Input: part model. Units: mm. Frame: model coordinates. A direction names the side the tool comes from. Give positions to 0.01 mm unless a question says otherwise; leave off trailing zeros. Loops run counter-clockwise (first coordinate to the right, second up) from the corner with the lowest first, then second, coordinate; pieces in that order, holes last. Notation, with made-up numbers: M 86,87 L 112,87 A12 cw 112,107 Z; hole C 17,21.25 d8. An arc over 180 degrees is marked long. Return JSON: item names as keys, results as strings. Group by question number.
```python
from build123d import *

# Parameters (mm, degrees)
CHAMFER1_SIZE                                    = 3.81
HOLE2_D                                          = 6
CIRPATTERN2_COUNT                                = 10
CBORE_FOR_1_4_SOCKET_SHOULDER_SCREW1_D           = 6.7564
CBORE_FOR_1_4_SOCKET_SHOULDER_SCREW1_CBORE_D     = 10.31748
CBORE_FOR_1_4_SOCKET_SHOULDER_SCREW1_CBORE_DEPTH = 4.7752
CIRPATTERN4_COUNT                                = 12
CUT_EXTRUDE3_REACH                               = 116.288
CIRPATTERN5_COUNT                                = 12


with BuildPart() as part:
    # Sketch1 → Revolve1 (revolve)
    with BuildSketch(Plane.XY):
        Polygon((79.375, 10.68578), (79.375, 17.03578), (13.52042, 17.03578), (13.52042, 25.13076), (9.71042, 25.13076), (9.71042, 0), (14.14526, -4.43484), (19.22526, -4.43484), (19.22526, 10.68578), align=None)
    revolve(axis=Axis((0, 0, 0), (0, 1, 0)))

    # Chamfer1
    chamfer1_edges = [part.edges().sort_by_distance(p)[0] for p in [
        (-13.52042, 25.13076, 0),
    ]]
    chamfer(chamfer1_edges, length=CHAMFER1_SIZE - 0.0001)  # a hair under: the kernel refuses the full size

    # Hole2 (through all)
    with Locations(Plane(origin=(0, 17.03578, 0), x_dir=(1, 0, 0), z_dir=(0, 1, 0))):
        with Locations((38.1, 0)):
            hole2 = Hole(HOLE2_D / 2)

    # CirPattern2: Hole2 ×10 about axis
    cirpattern2_axis = Axis((0, 0, 0), (0, 1, 0))
    for i in range(1, CIRPATTERN2_COUNT):
        add(hole2.rotate(cirpattern2_axis, i * 360 / CIRPATTERN2_COUNT), mode=Mode.SUBTRACT)

    # CBORE for 1/4 Socket Shoulder Screw1 (through all)
    with Locations(Plane(origin=(0, 17.03578, 0), x_dir=(1, 0, 0), z_dir=(0, 1, 0))):
        with Locations((72.39, 0)):
            cbore_for_1_4_socket_shoulder_screw1 = CounterBoreHole(CBORE_FOR_1_4_SOCKET_SHOULDER_SCREW1_D / 2, CBORE_FOR_1_4_SOCKET_SHOULDER_SCREW1_CBORE_D / 2, CBORE_FOR_1_4_SOCKET_SHOULDER_SCREW1_CBORE_DEPTH)

    # CirPattern4: CBORE for 1/4 Socket Shoulder Screw1 ×12 about axis
    cirpattern4_axis = Axis((0, 0, 0), (0, 1, 0))
    for i in range(1, CIRPATTERN4_COUNT):
        add(cbore_for_1_4_socket_shoulder_screw1.rotate(cirpattern4_axis, i * 360 / CIRPATTERN4_COUNT), mode=Mode.SUBTRACT)

    # Sketch17 → Cut-Extrude3 (cut, up to next)
    with BuildSketch(Plane(origin=(0, 17.03578, 0), x_dir=(1, 0, 0), z_dir=(0, 1, 0)), mode=Mode.PRIVATE) as cut_extrude3_sk1:
        with BuildLine():
            ThreePointArc((79.375, 0), (77.717548697, 4.517460557), (73.531778846, 6.891049707))
            ThreePointArc((73.531778846, 6.891049707), (68.521982999, 9.388428721), (65.780227273, 14.268770092))
            ThreePointArc((65.780227273, 14.268770092), (65.016467368, 17.421109926), (64.101732931, 20.532996256))
            ThreePointArc((64.101732931, 20.532996256), (64.035992356, 26.130373726), (67.12591332, 30.798065318))
            ThreePointArc((67.12591332, 30.798065318), (69.56410177, 34.946538746), (68.740766425, 39.6875))
            ThreePointArc((68.740766425, 39.6875), (76.670362462, 20.543761705), (79.375, 0))
        make_face()
    cut_extrude3_tool1 = extrude(cut_extrude3_sk1.sketch, amount=-CUT_EXTRUDE3_REACH, mode=Mode.PRIVATE) & part.part
    cut_extrude3 = cut_extrude3_tool1.solids().sort_by_distance((71.346501, 17.03578, -19.117237))[0]
    add(cut_extrude3, mode=Mode.SUBTRACT)

    # CirPattern5: Cut-Extrude3 ×12 about axis
    cirpattern5_axis = Axis((0, 0, 0), (0, 1, 0))
    for i in range(1, CIRPATTERN5_COUNT):
        add(cut_extrude3.rotate(cirpattern5_axis, i * 360 / CIRPATTERN5_COUNT), mode=Mode.SUBTRACT)


solid = part.part
```
Item 1: Section A-A, the plane z = 36.5. Return loops of the section in (x, y).
Item 2: Section B-B, the plane y = 3.75. Return loops of the section in (x, z).
Item 3: Reachability of faces 1 (the face through (-36.9, 14.7, -67.8)), 2 (the face through (-9.334, 13.905, -68.58)), 3 (the face through (4.481, 12.389, 8.615)), 4 (the face through (26, 14, 64)), 5 (the face through (68.58, 13.905, -9.334)) from +Z, -Z, +X, -X, +Y, -Y: full face, straight path, thin tool, end or side. Return the list, or none.
Item 4: First-contact query: pin 1 Ø6 at (y, z) = (21, -3.5) entering from +X; pin 2 Ø10 at (x, z) = (53.5, 2) entering from -Y; pin 3 Ø11.5 at (x, z) = (-73.5, 1.5) entering from +Y; pin 4 Ø6 at (x, z) = (0, 72.39) entering from +Y. Flat tips, straight axial feed; report the tip coordinate or a pass-through.
Item 5: Pull-direction query (X, two-part tool) for faces 6 (the face through (-67.04, 14.68, 33.42)), 7 (the face through (47.56, 13.91, 47.63)), 8 (the face through (-47.63, 13.91, 47.56)); classes: pulls with the +X half, pulls with the -X half, needs draft (parallel to the pull), parting line crosses it, or undercut.
Item 6: Material intervals for line 1 (Z direction, x = -38.1, y = 15.25); line 2 (X direction, y = 11.5, z = -20.5); line 3 (Z direction, x = -59.5, y = 16.75), sorted ascending. Write a range as from..to.
Answer below:
{
 "1": {"outline": "M -69.67,10.69 L -66.06,10.69 L -66.06,12.26 L -67.84,12.26 L -67.84,17.04 L -69.67,17.04 Z; M -59.33,10.69 L -14.76,10.69 L -14.76,17.04 L -57.54,17.04 L -57.54,12.26 L -59.33,12.26 Z; M -8.79,10.69 L 8.79,10.69 L 8.79,17.04 L -8.79,17.04 Z; M 14.76,10.69 L 59.33,10.69 L 59.33,12.26 L 57.54,12.26 L 57.54,17.04 L 14.76,17.04 Z; M 66.06,10.69 L 69.67,10.69 L 69.67,17.04 L 67.84,17.04 L 67.84,12.26 L 66.06,12.26 Z"},
 "2": {"outline": "C 0,0 d38.45; hole C 0,0 d19.42"},
 "3": {"face 1": "+Y", "face 2": "-Z, +Y, -Y", "face 3": "+Y, -Y", "face 4": "+Z, +Y, -Y", "face 5": "+X, +Y, -Y"},
 "4": {"pin 1": "x = 13.51", "pin 2": "y = 10.69", "pin 3": "y = 17.04", "pin 4": "through"},
 "5": {"face 6": "undercut", "face 7": "pulls with the +X half", "face 8": "pulls with the -X half"},
 "6": {"line 1": "-69.41..-67.49, -57.9..-3, 3..57.9, 67.49..69.41", "line 2": "-64.11..-33.15, -28.5..28.5, 33.15..64.11", "line 3": "-42.49..-40.25, -32.14..32.14, 40.25..42.49"}
}
